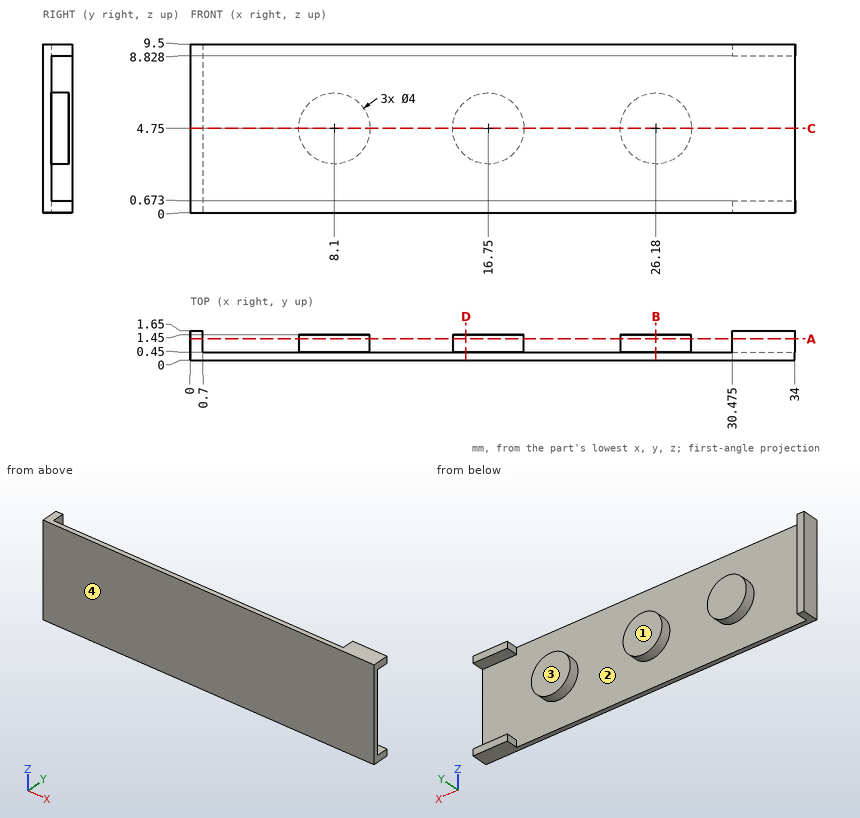
Here's the drawing with two shaded views (mm, measured from the low corner). I have some questions. A direction names the side the tool comes from. Coordinates: 2 decimals unless noted, no trailing zeros. Loops run counter-clockwise (first coordinate to the right, second up) from the corner with the lowest first, then second, coordinate; pieces in that order, holes last. Notation, with made-up numbers: M -15,-14 L 27,-14 A20 cw 27,15 Z; hole C -34,-5.5 d9. An arc over 180 degrees is marked long. Put each result on its own line as item: value. Start each with the question number.
(1) Imagine slicing it at B-B on x = 26.18. List the corners of the cut face in (y, z) for me.
(2) Will these pins go through, and if not, where does the flat tip stop? pin 1 Ø5 at (x, z) = (9, 3.5) entering from -Y; pin 2 Ø3 at (x, z) = (17, 4.5) entering from +Y; pin 3 Ø1.5 at (x, z) = (13, 4) entering from +Y.
(3) Imagine slicing it at D-D on x = 15.5. List the corners of the cut face in (y, z) for me.
(4) Which directions (+Z, -Z, +X, -X, +Y, -Y) give clear straight access to the entire face, cutting with the end or side of a thin tool? Please do the marked faces 3 and 4.
(5) Imagine slicing it at A-A on y = 1.2. Give the number of separate pieces and of enclosed holes in the cut face.
(6) I need wall thicknesses on probe 1 along X at (y, z) = (1.4, 5) (1 decimal); probe 2 along X at (y, z) = (1, 3.5); probe 3 along Y at (x, z) = (23, 3.5). Which ranges of each line are inside material? Lowest first, please.
(7) Imagine slicing it at C-C on z = 4.75. List the corners of the cut face in (x, y) for me.
(8) We'd pull the mould along X, two halves only. Please class the marked faces 1 and 2: +X half, -X half, draft (parallel to the pull), parting line (faces both ways), or undercut.
Worked answers:
1. outline: M 0,0 L 0.45,0 L 0.45,2.75 L 1.45,2.75 L 1.45,6.75 L 0.45,6.75 L 0.45,9.5 L 0,9.5 Z
2. pin 1: stops at y = 0
2. pin 2: stops at y = 1.45
2. pin 3: stops at y = 0.45
3. outline: M 0,0 L 0.45,0 L 0.45,3.19 L 1.45,3.19 L 1.45,6.31 L 0.45,6.31 L 0.45,9.5 L 0,9.5 Z
4. face 3: +Z, -Z, +X, +Y
4. face 4: +Z, -Z, +X, -X, -Y
5. separate pieces: 6
5. enclosed holes: 0
6. probe 1: x = 0 to 0.7, 6.1 to 10.1, 14.8 to 18.7, 24.2 to 28.2
6. probe 2: x = 0 to 0.7, 6.54 to 9.66, 15.19 to 18.31, 24.62 to 27.74
6. probe 3: y = 0 to 0.45
7. outline: M 0,0 L 34,0 L 34,0.45 L 28.18,0.45 L 28.18,1.45 L 24.18,1.45 L 24.18,0.45 L 18.75,0.45 L 18.75,1.45 L 14.75,1.45 L 14.75,0.45 L 10.1,0.45 L 10.1,1.45 L 6.1,1.45 L 6.1,0.45 L 0.7,0.45 L 0.7,1.65 L 0,1.65 Z
8. face 1: draft
8. face 2: undercut
